Geometry: final body of the model. Coordinates: model frame, mm. Face numbers are marked on the shaded views. A direction names the side the tool comes from. Give positions to 0.01 mm unless a question says otherwise; leave off trailing zeros. Order: outer loops, then holes, each group sorted by start corner. A loop starts at its lowest first (then second) coordinate and runs counter-clockwise, first axis right, second up. Notation, with made-up numbers: (-7, 83.5) -> (11, 83.5) arc R30 cw to (11, 112.5) -> close; hole circle Ø11 at (44.25, -38). An arc over 180 degrees is marked (long way). Answer in a Markdown table with one row per item. Add a question column.
Q1. Line query: line 1 along Y through (x, z) = (15.5, 4); line 2 along Z through (x, y) = (4.5, 1). Output: solid intervals per line, ascending. Write a range as from..to.
Q2. Contact query for flat-ended pins moving along their axis: P1, Ø4, axis at x = 2, z = -9.5, coming from the +Y side; P2, Ø1.5, axis at y = -0.5, z = -4, coming from the +X side; P3, Ø4, axis at x = -16.5, y = -5, coming from the -Z side. Output: stop coordinate, or through.
Q3. Set-up query: the marked faces 1 and 2. Return all of +Z, -Z, +X, -X, +Y, -Y with unobstructed straight access to the full face (end or side cutting, diameter ignored); none if empty.
Q4. Cut plane A-A on z = 8.5. Return the cut outline in (x, y), and give its area (3 significant figures).
Q5. Cut plane D-D on x = 13.5. Return the cut outline in (y, z).
Q6. Cut plane B-B on y = 0. Return the cut outline in (x, z), and give its area (3 significant figures).
Q7. Cut plane C-C on z = 26.5. Return the cut outline in (x, y), and give its area (3 significant figures).
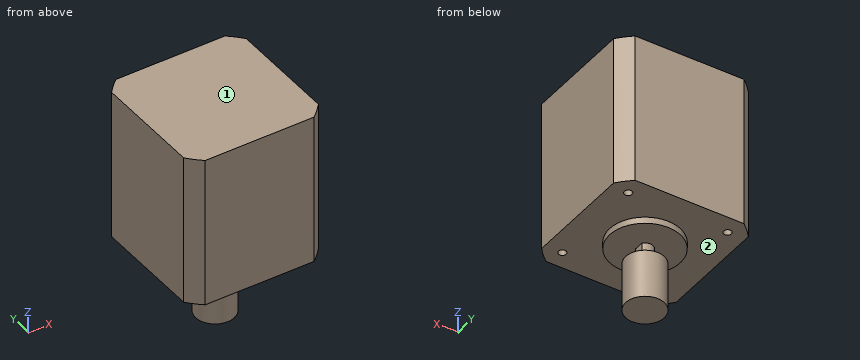
from build123d import *

# Parameters (mm, degrees)
F1_DEPTH = 47
F2_R     = 11
F3_DEPTH = 2
F4_D     = 2.4
F4_DEPTH = 13.8
F4_TIP   = 0.7210327428
F6_DEPTH = 20
F7_R     = 6
F8_DEPTH = 15


with BuildPart() as f1:
    # F0 (on Top) → F1 (new body)
    with BuildSketch(Plane.XY):
        with BuildLine():
            ThreePointArc((21, 16.9705627485), (19.091883092, 19.091883092), (16.9705627485, 21))
            Line((16.9705627485, 21), (-16.9705627485, 21))
            ThreePointArc((-16.9705627485, 21), (-19.091883092, 19.091883092), (-21, 16.9705627485))
            Line((-21, 16.9705627485), (-21, -16.9705627485))
            ThreePointArc((-21, -16.9705627485), (-19.091883092, -19.091883092), (-16.9705627485, -21))
            Line((-16.9705627485, -21), (16.9705627485, -21))
            ThreePointArc((16.9705627485, -21), (19.091883092, -19.091883092), (21, -16.9705627485))
            Line((21, -16.9705627485), (21, 16.9705627485))
        make_face()
    extrude(amount=F1_DEPTH)

    # F2 (on face) → F3 (join)
    with BuildSketch(Plane(origin=(0, 0, 0), x_dir=(1, 0, 0), z_dir=(0, 0, -1))):
        Circle(F2_R)
    extrude(amount=F3_DEPTH)

    # F4
    with Locations(Plane(origin=(0, 0, 0), x_dir=(1, 0, 0), z_dir=(0, 0, -1))):
        with Locations((-15.5, 15.5), (15.5, 15.5), (15.5, -15.5), (-15.5, -15.5)):
            Hole(F4_D / 2, depth=F4_DEPTH)
            with Locations((0, 0, -(F4_DEPTH + F4_TIP / 2))):  # 118° drill point
                Cone(0, F4_D / 2, F4_TIP, mode=Mode.SUBTRACT)

    # F5 (on face) → F6 (join)
    with BuildSketch(Plane(origin=(0, 0, -2), x_dir=(1, 0, 0), z_dir=(0, 0, -1))):
        with BuildLine():
            Line((2, -1.5), (2, 1.5))
            ThreePointArc((2, 1.5), (-2.5, 0), (2, -1.5))
        make_face()
    extrude(amount=F6_DEPTH)

    # F7 (on face) → F8 (join)
    with BuildSketch(Plane(origin=(0, 0, -22), x_dir=(1, 0, 0), z_dir=(0, 0, -1))):
        Circle(F7_R)
    extrude(amount=-F8_DEPTH)


solid = f1.part
Completed:
| question | item | result |
|---|---|---|
| 1 | line 1 | y = -21..-16.7, -14.3..14.3, 16.7..21 |
| 1 | line 2 | z = -22..-7, -2..47 |
| 2 | P1 | stops at y = 6 |
| 2 | P2 | stops at x = 2 |
| 2 | P3 | stops at z = 0 |
| 3 | face 1 | +Z, +X, -X, +Y, -Y |
| 3 | face 2 | -Z |
| 4 | outline | (-21, -16.97) arc R27 ccw to (-16.97, -21) -> (16.97, -21) arc R27 ccw to (21, -16.97) -> (21, 16.97) arc R27 ccw to (16.97, 21) -> (-16.97, 21) arc R27 ccw to (-21, 16.97) -> close; hole circle Ø2.4 at (-15.5, -15.5); hole circle Ø2.4 at (-15.5, 15.5); hole circle Ø2.4 at (15.5, -15.5); hole circle Ø2.4 at (15.5, 15.5) |
| 4 | area | 1,720 mm² |
| 5 | outline | (-21, 0) -> (21, 0) -> (21, 47) -> (-21, 47) -> close |
| 6 | outline | (-21, 0) -> (-11, 0) -> (-11, -2) -> (-2.5, -2) -> (-2.5, -7) -> (-6, -7) -> (-6, -22) -> (6, -22) -> (6, -7) -> (2, -7) -> (2, -2) -> (11, -2) -> (11, 0) -> (21, 0) -> (21, 47) -> (-21, 47) -> close |
| 6 | area | 2,220 mm² |
| 7 | outline | (-21, -16.97) arc R27 ccw to (-16.97, -21) -> (16.97, -21) arc R27 ccw to (21, -16.97) -> (21, 16.97) arc R27 ccw to (16.97, 21) -> (-16.97, 21) arc R27 ccw to (-21, 16.97) -> close |
| 7 | area | 1,730 mm² |
